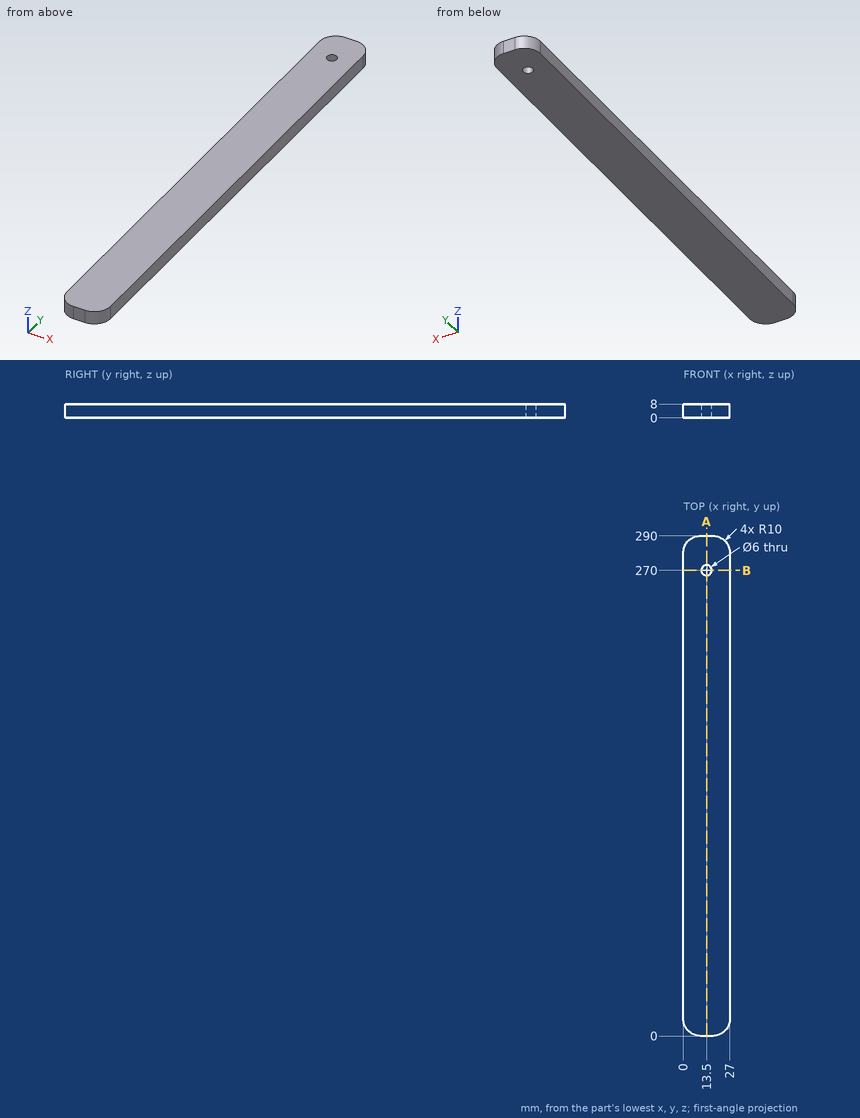
Drawing for the job (mm, zero at the part's lowest x, y, z). Give positions to 0.01 mm unless a question says otherwise; leave off trailing zeros. Loops run counter-clockwise (first coordinate to the right, second up) from the corner with the lowest first, then second, coordinate; pieces in that order, holes last. Notation, with made-up numbers: (-6, 29) - (52, 29) arc R31 ccw to (52, 60) - close; hole circle Ø6 at (14, 49.5). An arc over 180 degrees is marked (long way). Write item = value, one per line. Start each with the question number.
1) Band-saw the part on B-B on y = 270. Give the cut face in (x, z).
2) Band-saw the part on A-A on x = 13.5. Give the cut face in (y, z).
3) Probe probe 1 along Y at (x, z) = (13.5, 2.5); probe 2 along X at (y, z) = (270, 2.25); probe 3 along Y at (x, z) = (14.25, 3.5). List the from-to ranges inside material, lowest first. Write a range as from..to.
4) Drop flat-ended pins along their axis: pin 1 Ø1.5 at (x, z) = (5, 5) entering from +Y; pin 2 Ø1.5 at (x, z) = (9, 3) entering from -Y. Give the stop position or say it passes through.
Final values:
q1.outline = (0, 0) - (10.5, 0) - (10.5, 8) - (0, 8) - close; (16.5, 0) - (27, 0) - (27, 8) - (16.5, 8) - close
q2.outline = (0, 0) - (267, 0) - (267, 8) - (0, 8) - close; (273, 0) - (290, 0) - (290, 8) - (273, 8) - close
q3.probe_1 = 0..267, 273..290
q3.probe_2 = 0..10.5, 16.5..27
q3.probe_3 = 0..267.1, 272.9..290
q4.pin_1 = 289.05
q4.pin_2 = 0
